Autodesk Fusion 360 part; units mm, degrees
sketch "Sketch1" plane through (0, 0, 0) normal (0, 0, 1) x (1, 0, 0)
  line L0 (63.875, -42.75) -> (-63.875, -42.75)
  line L1 (-63.875, -42.75) -> (-63.875, 42.75)
  line L2 (-63.875, 42.75) -> (63.875, 42.75)
  line L3 (63.875, 42.75) -> (63.875, -42.75)
  line L4 (63.875, -42.75) -> (-63.875, 42.75) construction
  line L5 (-63.875, -42.75) -> (63.875, 42.75) construction
  dimension "d1" = 127.75
  dimension "d2" = 85.5
extrude "Extrude1" add sketch "Sketch1" along normal blind 3
sketch "Sketch2" plane through (0, 0, 3) normal (0, 0, 1) x (-1, 0, 0)
  line L0 (-63.875, -42.75) -> (63.875, -42.75)
  line L1 (63.875, -42.75) -> (63.875, 42.75)
  line L2 (63.875, 42.75) -> (-63.875, 42.75)
  line L3 (-63.875, 42.75) -> (-63.875, -42.75)
  line L4 (-63.875, -42.75) -> (-63.875, 42.75)
  line L5 (-63.875, 42.75) -> (63.875, 42.75)
  line L6 (63.875, 42.75) -> (63.875, -42.75)
  line L7 (63.875, -42.75) -> (-63.875, -42.75)
  line L8 (0, 0) -> (47.5, 0) construction
  line L9 (47.5, 0) -> (47.5, -22.5) construction
  circle A0 centre (47.5, -22.5) radius 13.5
  circle A1 centre (47.5, -22.5) radius 14
  circle A2 centre (15.8333, -22.5) radius 14
  circle A3 centre (-15.8333, -22.5) radius 14
  circle A4 centre (-47.5, -22.5) radius 14
  circle A5 centre (47.5, 22.5) radius 14
  circle A6 centre (15.8333, 22.5) radius 14
  circle A7 centre (-15.8333, 22.5) radius 14
  circle A8 centre (-47.5, 22.5) radius 14
  dimension "d5" = 47.5
  dimension "d6" = 22.5
  dimension "d7" = 27
  dimension "d8" = 0.5
  dimension "d15" = -95
  dimension "d16" = 45
extrude "Extrude2" add sketch "Sketch2" along normal blind 15 contours L0 L1 L2 L3 L4 L5 L6 L7
Source: CAD feature listing. Evaluate the final solid. Frame: model axes, mm. A direction names the side the tool comes from. Round coordinates to 2 decimals unless told otherwise and drop trailing zeros. Loops run counter-clockwise (first coordinate to the right, second up) from the corner with the lowest first, then second, coordinate; pieces in that order, holes last. Notation, with made-up numbers: (-19.75, 3.5) - (16.25, 3.5) arc R14 ccw to (16.25, 25.5) - close; hole circle Ø8 at (50.5, -25.75). An arc over 180 degrees is marked (long way). Write item = value, one per line. Start each with the question number.
(1) Set-up query: faces 4 (the face through (1, -42.75, 9)), 5 (the face through (-16, -22, 3)). Return all of +Z, -Z, +X, -X, +Y, -Y with unobstructed straight access to the full face (end or side cutting, diameter ignored); none if empty.
(2) Pull-direction query (X, two-part tool) for faces 1 (the face through (58.61, -31.02, 10.4)), 2 (the face through (63.875, 1, 9)), 3 (the face through (1, -1, 18)); classes: +X half, -X half, draft (parallel to the pull), parting line (faces both ways), or undercut.
(3) Ray query, line 1 along X through (y, z) = (22.5, 10.75) (3 decimals); line 2 along Y through (x, z) = (-47.5, 13.5); line 3 along X through (y, z) = (-13.5, 7.75) (1 decimal). Return the intervals inside material, ascending. Write a range as from..to.
(4) Section query C-C, the plane y = -22.5. Output: boundary loops of the cut face in (x, z) (3 decimals).
(5) Section query A-A, the plane z = 14.5. State how many separate pieces and enclosed holes the cut face has, plus the area to 3 significant figures.
(6) Section query D-D, the plane x = -26. Output: boundary loops of the cut face in (y, z), plus the area to 3 significant figures.
(7) Pin query (flat end, axial travel): pin 1 (14 mm diameter, centred on x = 14.5, y = -17, fed in from +Z). Return the tip coordinate at first contact, or that it passes through.
(8) Section query B-B, the plane x = 47.5. Output: boundary loops of the cut face in (y, z).
Conclusion:
q1.face_4 = +Z, -Z, +X, -X, -Y
q1.face_5 = +Z
q2.face_1 = undercut
q2.face_2 = +X half
q2.face_3 = draft
q3.line_1 = -63.875..-61.5, -33.5..-29.833, -1.833..1.833, 29.833..33.5, 61.5..63.875
q3.line_2 = -42.75..-36.5, -8.5..8.5, 36.5..42.75
q3.line_3 = -63.9..-58.2, -36.8..-26.6, -5.1..5.1, 26.6..36.8, 58.2..63.9
q4.outline = (-63.875, 0) - (63.875, 0) - (63.875, 18) - (61.5, 18) - (61.5, 3) - (33.5, 3) - (33.5, 18) - (29.833, 18) - (29.833, 3) - (1.833, 3) - (1.833, 18) - (-1.833, 18) - (-1.833, 3) - (-29.833, 3) - (-29.833, 18) - (-33.5, 18) - (-33.5, 3) - (-61.5, 3) - (-61.5, 18) - (-63.875, 18) - close
q5.separate_pieces = 1
q5.enclosed_holes = 8
q5.area = 6,000 mm2
q6.outline = (-42.75, 0) - (42.75, 0) - (42.75, 18) - (32.12, 18) - (32.12, 3) - (12.88, 3) - (12.88, 18) - (-12.88, 18) - (-12.88, 3) - (-32.12, 3) - (-32.12, 18) - (-42.75, 18) - close
q6.area = 962 mm2
q7.pin_1 = 3
q8.outline = (-42.75, 0) - (42.75, 0) - (42.75, 18) - (36.5, 18) - (36.5, 3) - (8.5, 3) - (8.5, 18) - (-8.5, 18) - (-8.5, 3) - (-36.5, 3) - (-36.5, 18) - (-42.75, 18) - close
